Read the model definition and answer for the solid it produces. Units are mm, in the model's axes. Coordinates: 2 decimals unless noted, no trailing zeros. Write each loop counter-clockwise with the first axis right and the second up, starting at its lowest first coordinate (ties: lowest second). Pieces come first, ordered by that corner, then holes. Notation, with made-up numbers: (-38, 78.5) -> (-33, 78.5) arc R32 ccw to (-33, 105.5) -> close; hole circle Ø8 at (48.25, 6). An arc over 180 degrees is marked (long way). One line per item, written item: value. Start each with the question number.
1. Consider line 1 along Z through (x, y) = (1.15, 7.5); line 2 along Y through (x, z) = (2, -0.75); line 3 along Y through (x, z) = (3, -3.25). Determine where each line is inside the solid, lowest interval first.
2. Find section C-C, the plane x = 0.9. Write down the section's boundary in (y, z).
3. Given P1, Ø1.6, axis at y = -7.5, z = 0, coming from the +X side (3 decimals), flat-ended and moving along its own axis, determine where the tip first touches the part or whether it passes through.
4. Find section D-D, the plane z = -5. Write down the section's boundary in (x, y) (3 decimals), and give its area (3 significant figures).
5. For a pull along Y with two mould halves and no side action, classify faces 1 (the flat face through (2, 15, 0)), 2 (the cylindrical face through (2, -99, -4)), 3 (the cylindrical face through (1.565, -3.746, 0.165)) as pulls with the +Y half, pulls with the -Y half, needs draft (parallel to the pull), parting line crosses it, or undercut.
6. Find section B-B, the plane z = 0. Write down the section's boundary in (x, y) (3 decimals).
7. Find section A-A, the plane y = -10.5. Write down the section's boundary in (x, z) (3 decimals), and give its area (4 significant figures).
```python
from build123d import *

# Parameters (mm, degrees)
F0_W     = 115
F0_H     = 12
F0_R     = 1
F0_R_2   = 3.75
F1_DEPTH = 3.175
F2_R     = 5
F3_R     = 5
F4_R     = 5
F5_R     = 5


# Not quite as in the source:
# - a length typed as a fraction of an inch, garbled in the dataset ("3 / 203.2 mm" for 3/8 in), is restored


with BuildPart() as f1:
    # F0 (on Right) → F1 (new body)
    with BuildSketch(Plane.YZ):
        with Locations((-42.5, 0)):
            Rectangle(F0_W, F0_H)
        with Locations((-10.5, 0)):
            Circle(F0_R, mode=Mode.SUBTRACT)
        with Locations((-7.5, 0)):
            Circle(F0_R, mode=Mode.SUBTRACT)
        Circle(F0_R_2, mode=Mode.SUBTRACT)
        with Locations((7.5, 0)):
            Circle(F0_R, mode=Mode.SUBTRACT)
        with Locations((10.5, 0)):
            Circle(F0_R, mode=Mode.SUBTRACT)
    extrude(amount=F1_DEPTH)

    # F2
    f2_edges = [f1.edges().sort_by_distance(p)[0] for p in [
        (1.5875, -100, 6),
    ]]
    fillet(f2_edges, radius=F2_R)

    # F3
    f3_edges = [f1.edges().sort_by_distance(p)[0] for p in [
        (1.5875, -100, -6),
    ]]
    fillet(f3_edges, radius=F3_R)

    # F4
    f4_edges = [f1.edges().sort_by_distance(p)[0] for p in [
        (1.5875, 15, 6),
    ]]
    fillet(f4_edges, radius=F4_R)

    # F5
    f5_edges = [f1.edges().sort_by_distance(p)[0] for p in [
        (1.5875, 15, -6),
    ]]
    fillet(f5_edges, radius=F5_R)


solid = f1.part
```
Answer block:
1. line 1: z = -6 to -1, 1 to 6
1. line 2: y = -100 to -11.16, -9.84 to -8.16, -6.84 to -3.67, 3.67 to 6.84, 8.16 to 9.84, 11.16 to 15
1. line 3: y = -99.47 to -1.87, 1.87 to 14.47
2. outline: (-100, -1) arc R5 ccw to (-95, -6) -> (10, -6) arc R5 ccw to (15, -1) -> (15, 1) arc R5 ccw to (10, 6) -> (-95, 6) arc R5 ccw to (-100, 1) -> close; hole circle Ø2 at (-10.5, 0); hole circle Ø2 at (-7.5, 0); hole circle Ø7.5 at (0, 0); hole circle Ø2 at (7.5, 0); hole circle Ø2 at (10.5, 0)
3. P1: passes through
4. outline: (0, -98) -> (3.175, -98) -> (3.175, 13) -> (0, 13) -> close
4. area: 352 mm2
5. face 1: pulls with the +Y half
5. face 2: pulls with the -Y half
5. face 3: undercut
6. outline: (0, -100) -> (3.175, -100) -> (3.175, -11.5) -> (0, -11.5) -> close; (0, -9.5) -> (3.175, -9.5) -> (3.175, -8.5) -> (0, -8.5) -> close; (0, -6.5) -> (3.175, -6.5) -> (3.175, -3.75) -> (0, -3.75) -> close; (0, 3.75) -> (3.175, 3.75) -> (3.175, 6.5) -> (0, 6.5) -> close; (0, 8.5) -> (3.175, 8.5) -> (3.175, 9.5) -> (0, 9.5) -> close; (0, 11.5) -> (3.175, 11.5) -> (3.175, 15) -> (0, 15) -> close
7. outline: (0, -6) -> (3.175, -6) -> (3.175, -1) -> (0, -1) -> close; (0, 1) -> (3.175, 1) -> (3.175, 6) -> (0, 6) -> close
7. area: 31.75 mm2
